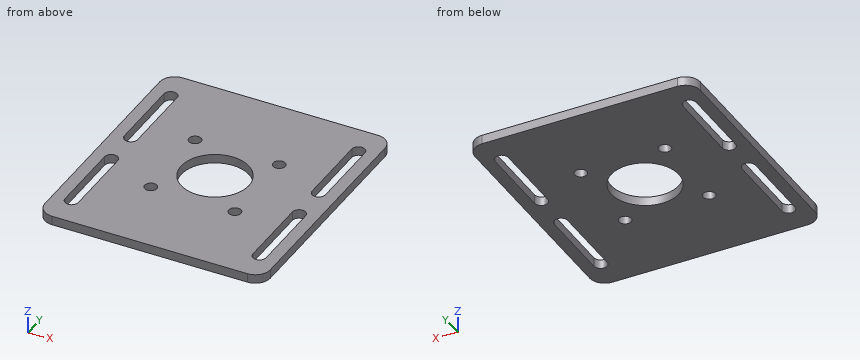
from build123d import *

# Parameters (mm, degrees)
SKETCH_1_W          = 300
SKETCH_1_H          = 330
SKETCH_1_R          = 45
EXTRUDE_1_DEPTH     = 6
FILLET_1_R          = 20
SKETCH_3_R          = 8.1
CUT_EXTRUDE_2_DEPTH = 12
CUT_EXTRUDE_3_DEPTH = 12


with BuildPart() as part:
    # Эскиз1 → Бобышка-Вытянуть1 (new, symmetric)
    with BuildSketch(Plane.XY):
        Rectangle(SKETCH_1_W, SKETCH_1_H)
        Circle(SKETCH_1_R, mode=Mode.SUBTRACT)
    extrude(amount=EXTRUDE_1_DEPTH, both=True)

    # Скругление1
    fillet_1_edges = [part.edges().sort_by_distance(p)[0] for p in [
        (150, -165, 0),
        (-150, -165, 0),
        (-150, 165, 0),
        (150, 165, 0),
    ]]
    fillet(fillet_1_edges, radius=FILLET_1_R)

    # Эскиз3 → Вырез-Вытянуть2 (cut)
    with BuildSketch(Plane.XY.offset(6)):
        with Locations((-56, 56)):
            Circle(SKETCH_3_R)
        with Locations((56, 56)):
            Circle(SKETCH_3_R)
        with Locations((56, -56)):
            Circle(SKETCH_3_R)
        with Locations((-56, -56)):
            Circle(SKETCH_3_R)
    extrude(amount=-CUT_EXTRUDE_2_DEPTH, mode=Mode.SUBTRACT)

    # Эскиз4 → Вырез-Вытянуть3 (cut)
    with BuildSketch(Plane(origin=(0, 0, -6), x_dir=(-1, 0, 0), z_dir=(0, 0, -1))):
        with BuildLine():
            Line((-133.8, 25), (-133.8, 125))
            ThreePointArc((-133.8, 125), (-125, 133.8), (-116.2, 125))
            Line((-116.2, 125), (-116.2, 25))
            ThreePointArc((-116.2, 25), (-125, 16.2), (-133.8, 25))
        make_face()
        with BuildLine():
            Line((-133.8, -25), (-133.8, -125))
            ThreePointArc((-133.8, -125), (-125, -133.8), (-116.2, -125))
            Line((-116.2, -125), (-116.2, -25))
            ThreePointArc((-116.2, -25), (-125, -16.2), (-133.8, -25))
        make_face()
        with BuildLine():
            Line((133.8, -25), (133.8, -125))
            ThreePointArc((133.8, -125), (125, -133.8), (116.2, -125))
            Line((116.2, -125), (116.2, -25))
            ThreePointArc((116.2, -25), (125, -16.2), (133.8, -25))
        make_face()
        with BuildLine():
            Line((133.8, 25), (133.8, 125))
            ThreePointArc((133.8, 125), (125, 133.8), (116.2, 125))
            Line((116.2, 125), (116.2, 25))
            ThreePointArc((116.2, 25), (125, 16.2), (133.8, 25))
        make_face()
    extrude(amount=-CUT_EXTRUDE_3_DEPTH, mode=Mode.SUBTRACT)


solid = part.part
Here's how the part is built. I have some questions about the finished solid (model axes, mm). Round coordinates to 2 decimals unless told otherwise and drop trailing zeros. Order: outer loops, then holes, each group sorted by start corner. A loop starts at its lowest first (then second) coordinate and runs counter-clockwise, first axis right, second up. Notation, with made-up numbers: (-20, 62.5) -> (34, 62.5) arc R14 cw to (34, 78.5) -> close; hole circle Ø5 at (-9, 8.5). An arc over 180 degrees is marked (long way). Use CSV: the item, a comma, the result in double quotes.
1. I want a section at D-D on z = -4. Give the number of separate pieces and of enclosed holes in the cut face, and give its area (3 significant figures).
Recorded:
separate pieces,"1"
enclosed holes,"9"
area,"83,500 mm2"
2. I'm going to push flat-ended pins straight in: P1, Ø14.5, axis at x = 56, y = -56, coming from the -Z side; P2, Ø18.5, axis at x = -56, y = 56, coming from the -Z side. Where does each tip first touch, or does it pass through?
Recorded:
P1,"passes through"
P2,"stops at z = -6"
3. I want a section at C-C on y = -105.5. List the corners of the cut face in (x, z) for me.
Recorded:
outline,"(-150, -6) -> (-133.8, -6) -> (-133.8, 6) -> (-150, 6) -> close; (-116.2, -6) -> (116.2, -6) -> (116.2, 6) -> (-116.2, 6) -> close; (133.8, -6) -> (150, -6) -> (150, 6) -> (133.8, 6) -> close"
4. I want a section at B-B on x = 56. List the corners of the cut face in (y, z) for me, and give its area (3 significant figures).
Recorded:
outline,"(-165, -6) -> (-64.1, -6) -> (-64.1, 6) -> (-165, 6) -> close; (-47.9, -6) -> (47.9, -6) -> (47.9, 6) -> (-47.9, 6) -> close; (64.1, -6) -> (165, -6) -> (165, 6) -> (64.1, 6) -> close"
area,"3,570 mm2"
5. I need wall thicknesses on line 1 along X through (y, z) = (74, 4.75); line 2 along Y through (x, z) = (-56, 3); line 3 along Y through (x, z) = (51.5, 2.25). Which ranges of each line are inside material? Lowest first, please.
Recorded:
line 1,"x = -150 to -133.8, -116.2 to 116.2, 133.8 to 150"
line 2,"y = -165 to -64.1, -47.9 to 47.9, 64.1 to 165"
line 3,"y = -165 to -62.73, -49.27 to 49.27, 62.73 to 165"
6. I want a section at A-A on y = 0. List the corners of the cut face in (x, z) for me, and give its area (3 significant figures).
Recorded:
outline,"(-150, -6) -> (-45, -6) -> (-45, 6) -> (-150, 6) -> close; (45, -6) -> (150, -6) -> (150, 6) -> (45, 6) -> close"
area,"2,520 mm2"
